Drawing for the job (mm, zero at the part's lowest x, y, z). Give positions to 0.01 mm unless a question says otherwise; leave off trailing zeros. Loops run counter-clockwise (first coordinate to the right, second up) from the corner with the lowest first, then second, coordinate; pieces in that order, holes last.
1) Band-saw the part on D-D on y = 2.5. List the corners of the cut face in (x, z) (3 decimals).
2) Band-saw the part on B-B on x = 6.25. List the corners of the cut face in (y, z) (3 decimals), then the cut area to 3 significant figures.
3) Band-saw the part on A-A on z = 6.25. List the corners of the cut face in (x, y) (3 decimals), then the cut area to 3 significant figures.
4) Flat gauge pins, fed straight in: P1, Ø1.5, axis at x = 9.5, y = 5, coming from the +Z side; P2, Ø6, axis at x = 7.5, z = 8, coming from the -Y side; P3, Ø6.5, axis at x = 6.25, z = 6.25, coming from the -Y side (3 decimals). Where does each tip first touch, or does it go through?
5) Two-plate mould, pull along X, no slides. Class the marked faces 1, 2, 3 and 4: +X half, -X half, draft (parallel to the pull), parting line (faces both ways), or undercut.
6) Wall check: line 1 (Y direction, x = 2.5, z = 11); line 2 (Z direction, x = 6.75, y = 6.5); line 3 (X direction, y = 4, z = 6.5). Give the ranges that are in metal, low to high.
7) Band-saw the part on C-C on y = 4.5. List the corners of the cut face in (x, z), then the cut area to 3 significant figures.
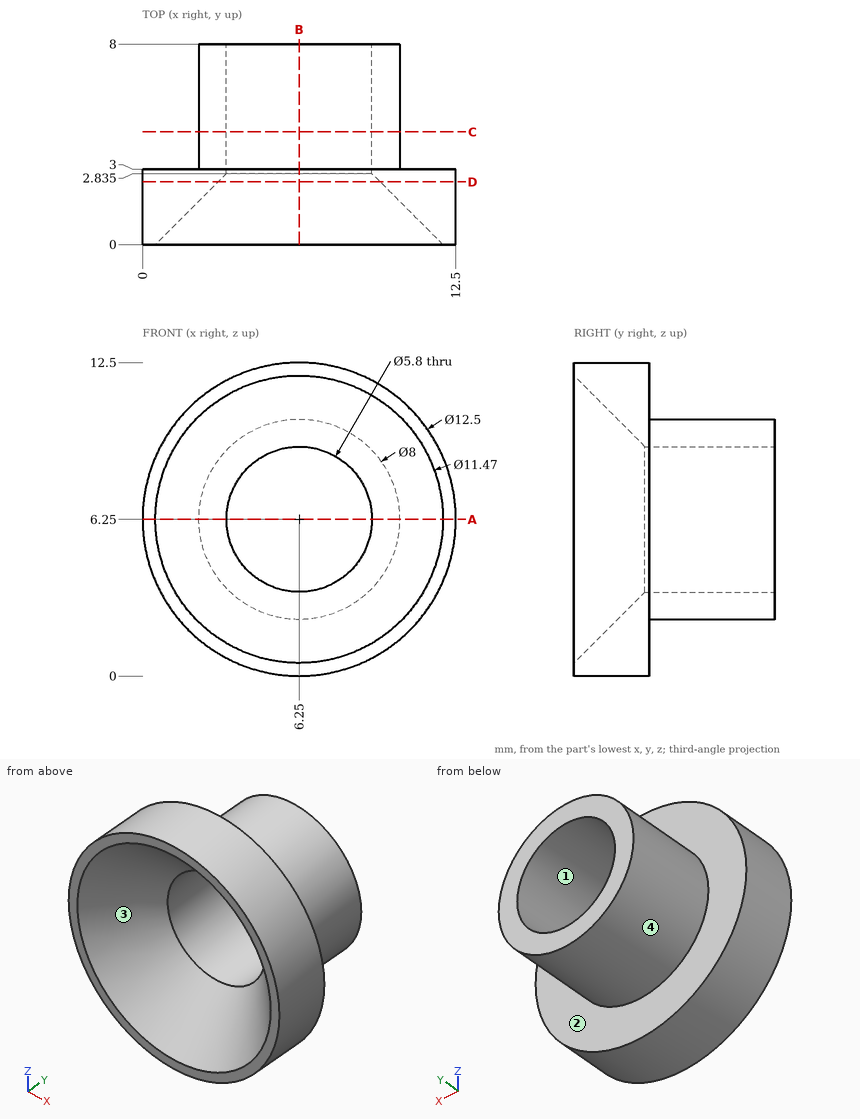
Findings below:
1. outline: circle Ø12.5 at (6.25, 6.25); hole circle Ø6.47 at (6.25, 6.25)
2. outline: (0, 0) - (3, 0) - (3, 2.25) - (8, 2.25) - (8, 3.35) - (2.835, 3.35) - (0, 0.515) - close; (0, 11.985) - (2.835, 9.15) - (8, 9.15) - (8, 10.25) - (3, 10.25) - (3, 12.5) - (0, 12.5) - close
2. area: 23.1 mm2
3. outline: (0, 0) - (0.515, 0) - (3.35, 2.835) - (3.35, 8) - (2.25, 8) - (2.25, 3) - (0, 3) - close; (9.15, 2.835) - (11.985, 0) - (12.5, 0) - (12.5, 3) - (10.25, 3) - (10.25, 8) - (9.15, 8) - close
3. area: 23.1 mm2
4. P1: stops at z = 9.37
4. P2: stops at y = 0.58
4. P3: stops at y = 2.485
5. face 1: undercut
5. face 2: draft
5. face 3: undercut
5. face 4: parting line
6. line 1: y = 0 to 3
6. line 2: z = 2.28 to 3.39, 9.11 to 10.22
6. line 3: x = 2.26 to 3.36, 9.14 to 10.24
7. outline: circle Ø8 at (6.25, 6.25); hole circle Ø5.8 at (6.25, 6.25)
7. area: 23.8 mm2
